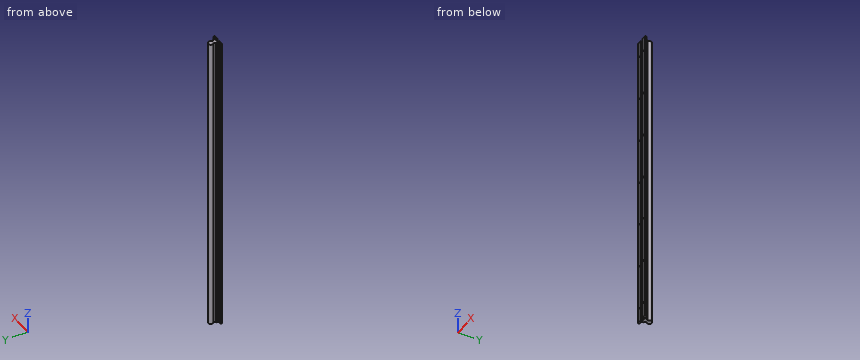
from build123d import *

# Parameters (mm, degrees)
BOSS_EXTRUDE1_DEPTH = 500
SKETCH2_R           = 2.75
CUT_EXTRUDE1_DEPTH  = 6
LPATTERN1_COUNT     = 7
LPATTERN1_PITCH     = 150


with BuildPart() as part:
    # Sketch1 → Boss-Extrude1 (new body, symmetric)
    with BuildSketch(Plane.XY):
        with BuildLine():
            Line((-7.008955797, -13.3), (-3.487119155, -7.2))
            ThreePointArc((-3.487119155, -7.2), (0, 8), (3.487119155, -7.2))
            Line((3.487119155, -7.2), (7.008955797, -13.3))
            Line((7.008955797, -13.3), (9.25, -13.3))
            Line((9.25, -13.3), (9.25, -20))
            Line((9.25, -20), (20, -20))
            Line((20, -20), (20, -25))
            Line((20, -25), (5, -25))
            Line((5, -25), (5, -19))
            Line((5, -19), (-5, -19))
            Line((-5, -19), (-5, -25))
            Line((-5, -25), (-20, -25))
            Line((-20, -25), (-20, -20))
            Line((-20, -20), (-9.25, -20))
            Line((-9.25, -20), (-9.25, -13.3))
            Line((-9.25, -13.3), (-7.008955797, -13.3))
        make_face()
    extrude(amount=BOSS_EXTRUDE1_DEPTH, both=True)

    # Sketch2 → Cut-Extrude1 (cut, through all)
    with BuildSketch(Plane(origin=(0, -20, 0), x_dir=(1, 0, 0), z_dir=(0, 1, 0))):
        with Locations(Location((15, -450, 0), (0, 0, 270))):  # turned: the seam where the file's is
            Circle(SKETCH2_R)
        with Locations(Location((-15, -450, 0), (0, 0, 270))):  # turned: the seam where the file's is
            Circle(SKETCH2_R)
    cut_extrude1 = extrude(amount=-CUT_EXTRUDE1_DEPTH, mode=Mode.SUBTRACT)

    # LPattern1: Cut-Extrude1 ×7
    with Locations(*[(0, 0, -i * LPATTERN1_PITCH) for i in range(1, LPATTERN1_COUNT)]):
        add(cut_extrude1, mode=Mode.SUBTRACT)


solid = part.part
Design review of the part built by this model. Coordinates are the model's own, in mm. Round coordinates to 2 decimals unless told otherwise and drop trailing zeros. Loops run counter-clockwise (first coordinate to the right, second up) from the corner with the lowest first, then second, coordinate; pieces in that order, holes last. Notation, with made-up numbers: (89, 57.5) - (125, 57.5) arc R15 cw to (125, 75.5) - close; hole circle Ø3 at (6.5, -22.5). An arc over 180 degrees is marked (long way). One line per question, with ' | ' between items.
1. We need section A-A, the plane z = -79.5. State the section outline as (x, y) points.
Results are:
outline: (-20, -25) - (-5, -25) - (-5, -19) - (5, -19) - (5, -25) - (20, -25) - (20, -20) - (9.25, -20) - (9.25, -13.3) - (7.01, -13.3) - (3.49, -7.2) arc R8 ccw (long way) to (-3.49, -7.2) - (-7.01, -13.3) - (-9.25, -13.3) - (-9.25, -20) - (-20, -20) - close
2. For L1, parallel to X at y = -23.9, z = -300; L2, parallel to X at y = -21, z = -9.5; L3, parallel to Y at x = -4.5, z = 450, list the stretches that pass through material, from the lowest coordinate up. Write a range as [from, to].
Results are:
L1: x = [-20, -17.75], [-12.25, -5], [5, 12.25], [17.75, 20] | L2: x = [-20, -5], [5, 20] | L3: y = [-19, -8.95], [-6.61, 6.61]
3. Clearance check with flat-ended pins moving along their axes: P1, Ø6.5, axis at x = 15, z = -450, coming from the -Y side; P2, Ø4.5, axis at x = 15, z = 0, coming from the -Y side; P3, Ø4, axis at x = 5.5, z = -392.5, coming from the +Y side; P4, Ø7, axis at x = 15, z = 450, coming from the +Y side. State where each tip first meets the part, or that it passes through.
Results are:
P1: stops at y = -25 | P2: passes through | P3: stops at y = 7.19 | P4: stops at y = -20
4. We need section B-B, the plane y = 0. State the section outline as (x, z) points.
Results are:
outline: (-8, -500) - (8, -500) - (8, 500) - (-8, 500) - close
